```python
from build123d import *

# Parameters (mm, degrees)
F1_DEPTH = 50
F3_DEPTH = 100


with BuildPart() as f1:
    # F0 (on Top) → F1 (new body)
    with BuildSketch(Plane.XY):
        Polygon((0, 100), (0, 0), (50, 100), align=None)
    extrude(amount=F1_DEPTH)

    # F2 (on Front) → F3 (join)
    with BuildSketch(Plane.XZ):
        Polygon((50, 0), (0, 49.431257), (0, 0), align=None)
    extrude(amount=-F3_DEPTH)


solid = f1.part
```
The listing builds one solid part. Answer for the finished solid, in the listing's coordinates (mm). A direction names the side the tool comes from. Give positions to 0.01 mm unless a question says otherwise; leave off trailing zeros. Order: outer loops, then holes, each group sorted by start corner. A loop starts at its lowest first (then second) coordinate and runs counter-clockwise, first axis right, second up.
Item 1: The part is cut by section A-A, the plane z = 43.5. Give the vertices of the cut face in (x, y), and give its area (3 significant figures).
From the geometry:
outline: (0, 0) - (6, 0) - (6, 12) - (50, 100) - (0, 100) - close
area: 2,540 mm2
Item 2: The part is cut by section B-B, the plane x = 45. Give the vertices of the cut face in (y, z), and give its area (3 significant figures).
From the geometry:
outline: (0, 0) - (100, 0) - (100, 50) - (90, 50) - (90, 4.94) - (0, 4.94) - close
area: 945 mm2
Item 3: The part is cut by section D-D, the plane x = 34.5. Give the vertices of the cut face in (y, z).
From the geometry:
outline: (0, 0) - (100, 0) - (100, 50) - (69, 50) - (69, 15.32) - (0, 15.32) - close
Item 4: Which of the six approach directions +Z, -Z, +X, -X, +Y, -Y give full straight-line access (tool end or side, diameter ignored) to faces 1 (the face through (30.906, 38.189, 18.877)), 2 (the face through (25, 49, 0))?
From the geometry:
face 1: +Z, +X, -Y
face 2: -Z, +X, -X, +Y, -Y
Item 5: The part is cut by section C-C, the plane y = 51.5. Give the vertices of the cut face in (x, z).
From the geometry:
outline: (0, 0) - (50, 0) - (25.75, 23.97) - (25.75, 50) - (0, 50) - close
Item 6: Given pin 1 Ø6 at (y, z) = (36, 37.5) entering from +X; pin 2 Ø1 at (y, z) = (54.5, 18) entering from +X; pin 3 Ø8 at (y, z) = (33.5, 30.5) entering from +X, each flat-ended and moving along its own axis, determine where each tip first touches the part or whether it passes through.
From the geometry:
pin 1: stops at x = 19.5
pin 2: stops at x = 32.3
pin 3: stops at x = 23.2
Item 7: Find the intervals of material crossed by probe 1 along Y at (x, z) = (12.5, 43.5); probe 2 along X at (y, z) = (39.5, 19); probe 3 along Z at (x, y) = (31.5, 17.5), in increasing order.
From the geometry:
probe 1: y = 25 to 100
probe 2: x = 0 to 30.78
probe 3: z = 0 to 18.29
